Read the model definition and answer for the solid it produces. Units are mm, in the model's axes. A direction names the side the tool comes from. Coordinates: 2 decimals unless noted, no trailing zeros. Loops run counter-clockwise (first coordinate to the right, second up) from the corner with the lowest first, then second, coordinate; pieces in that order, holes last. Notation, with made-up numbers: M 51,-31 L 110,-31 A31 ccw 110,-5 Z; hole C 81,-32 d6. An arc over 180 degrees is marked long. Put each result on its own line as item: value.
from build123d import *

# Parameters (mm, degrees)
BOSS_EXTRUDE1_DEPTH     = 3.175
SKETCH2_R               = 19.9
CUT_EXTRUDE1_DEPTH      = 140.49939292
ESQUISSE2_R             = 1.5
ENL_V_MAT_EXTRU_1_DEPTH = 140.49939292
SKETCH5_R               = 1.625
CUT_EXTRUDE3_DEPTH      = 140.49939292
CUT_EXTRUDE4_DEPTH      = 140.49939292


with BuildPart() as part:
    # Sketch1 → Boss-Extrude1 (new body)
    with BuildSketch(Plane(origin=(0, 0, 0), x_dir=(1, 0, 0), z_dir=(0, 1, 0))):
        with BuildLine():
            Line((-27.5, -100), (-34.975254116, 98.684097441))
            ThreePointArc((-34.975254116, 98.684097441), (0, 135), (34.975254116, 98.684097441))
            Line((34.975254116, 98.684097441), (27.5, -100))
            ThreePointArc((27.5, -100), (0, -127.5), (-27.5, -100))
        make_face()
    extrude(amount=BOSS_EXTRUDE1_DEPTH)

    # Sketch2 → Cut-Extrude1 (cut, through all)
    with BuildSketch(Plane(origin=(0, 3.175, 0), x_dir=(1, 0, 0), z_dir=(0, 1, 0))):
        with Locations(Location((0, -100, 0), (0, 0, 270))):
            Circle(SKETCH2_R)
        with Locations(Location((0, 100, 0), (0, 0, 270))):
            Circle(SKETCH2_R)
    extrude(amount=-CUT_EXTRUDE1_DEPTH, mode=Mode.SUBTRACT)

    # Esquisse2 → Enlèv. mat.-Extru.1 (cut, through all)
    with BuildSketch(Plane(origin=(0, 3.175, 0), x_dir=(1, 0, 0), z_dir=(0, 1, 0))):
        with Locations(Location((19.339370465, 80.660629535, 0), (0, 0, 270))):
            Circle(ESQUISSE2_R)
        with Locations(Location((19.339370465, 119.339370465, 0), (0, 0, 270))):
            Circle(ESQUISSE2_R)
        with Locations(Location((-19.339370465, 119.339370465, 0), (0, 0, 270))):
            Circle(ESQUISSE2_R)
        with Locations(Location((-19.339370465, 80.660629535, 0), (0, 0, 270))):
            Circle(ESQUISSE2_R)
    extrude(amount=-ENL_V_MAT_EXTRU_1_DEPTH, mode=Mode.SUBTRACT)

    # Sketch5 → Cut-Extrude3 (cut, through all)
    with BuildSketch(Plane(origin=(0, 3.175, 0), x_dir=(1, 0, 0), z_dir=(0, 1, 0))):
        with Locations(Location((-27.256476824, 42.340455159, 0), (0, 0, 270))):
            Circle(SKETCH5_R)
        with Locations(Location((-26.241351992, 15.359544841, 0), (0, 0, 270))):
            Circle(SKETCH5_R)
        with Locations(Location((26.241351992, 15.359544841, 0), (0, 0, 270))):
            Circle(SKETCH5_R)
        with Locations(Location((27.256476824, 42.340455159, 0), (0, 0, 270))):
            Circle(SKETCH5_R)
        Polygon((-21.15, 45.828069991), (-16.978069991, 50), (16.978069991, 50), (21.15, 45.828069991), (21.15, 11.871930009), (16.978069991, 7.7), (-16.978069991, 7.7), (-21.15, 11.871930009), align=None)
    extrude(amount=-CUT_EXTRUDE3_DEPTH, mode=Mode.SUBTRACT)

    # Sketch7 → Cut-Extrude4 (cut, through all)
    with BuildSketch(Plane(origin=(0, 3.175, 0), x_dir=(1, 0, 0), z_dir=(0, 1, 0))):
        with BuildLine():
            Line((17.892039301, -34.947326615), (-12.749738424, -9.235822228))
            ThreePointArc((-12.749738424, -9.235822228), (-18.385066635, -9.728849561), (-17.892039301, -15.364177772))
            Line((-17.892039301, -15.364177772), (12.749738424, -41.07568216))
            ThreePointArc((12.749738424, -41.07568216), (18.385066635, -40.582654826), (17.892039301, -34.947326615))
        make_face()
    extrude(amount=-CUT_EXTRUDE4_DEPTH, mode=Mode.SUBTRACT)


solid = part.part
1) Find section B-B, the plane z = 12.3. Write down the section's boundary in (x, y) (3 decimals), plus the area to 3 significant figures.
Answer list:
outline: M -30.8,0 L -19.321,0 L -19.321,3.175 L -30.8,3.175 Z; M -9.098,0 L 30.8,0 L 30.8,3.175 L -9.098,3.175 Z
area: 163 mm^2
2) Which of the six approach directions +Z, -Z, +X, -X, +Y, -Y give full straight-line access (tool end or side, diameter ignored) to faces 1 (the flat face through (-2.786, 1.61, 28.04)), 2 (the flat face through (-31.185, 1.565, 2.049))?
Answer list:
face 1: +Y, -Y
face 2: +Z, -X, +Y, -Y
3) Find section A-A, the plane x = 0. Write down the section's boundary in (y, z) (3 decimals).
Answer list:
outline: M 0,-135 L 3.175,-135 L 3.175,-119.9 L 0,-119.9 Z; M 0,-80.1 L 3.175,-80.1 L 3.175,-50 L 0,-50 Z; M 0,-7.7 L 3.175,-7.7 L 3.175,19.934 L 0,19.934 Z; M 0,30.377 L 3.175,30.377 L 3.175,80.1 L 0,80.1 Z; M 0,119.9 L 3.175,119.9 L 3.175,127.5 L 0,127.5 Z
4) Straight lines are drawn through the part: line 1 (Z direction, x = -9, y = 0.9); line 2 (Z direction, x = -11, y = 1.65); line 3 (X direction, y = 2.45, z = 100). For each, find the intervals that lie inside material, in ascending order. Write a range as [from, to].
Answer list:
line 1: z = [-133.82, -117.75], [-82.25, -50], [-7.7, 12.38], [22.83, 82.25], [117.75, 125.99]
line 2: z = [-133.23, -116.58], [-83.42, -50], [-7.7, 10.7], [21.15, 83.42], [116.58, 125.2]
line 3: x = [-27.5, -19.9], [19.9, 27.5]
5) Find section D-D, the plane z = -29. Write down the section's boundary in (x, y) (3 decimals).
Answer list:
outline: M -32.353,0 L -21.15,0 L -21.15,3.175 L -32.353,3.175 Z; M 21.15,0 L 32.353,0 L 32.353,3.175 L 21.15,3.175 Z
6) Given pin 1 Ø1.6 at (y, z) = (1, -35) entering from -X; pin 2 Ø1 at (y, z) = (1, -97.5) entering from -X; pin 3 Ø1 at (y, z) = (2, -65.5) entering from -X, each flat-ended and moving along its own axis, determine where each tip first touches the part or whether it passes through.
Answer list:
pin 1: stops at x = -32.61
pin 2: stops at x = -34.95
pin 3: stops at x = -33.75
7) Find section C-C, the plane y = 1.45. Count the separate pieces of the cut face and the enclosed holes in it, plus the area to 3 significant figures.
Answer list:
separate pieces: 1
enclosed holes: 12
area: 10,900 mm^2
8) Determine the mould class of faces 3 (the flat face through (31.29, 1.57, -0.73)), 4 (the cylindrical face through (-12.1, 1.6, 84.2)), 5 (the flat face through (0, 3.175, -6)) for opening direction X: released by +X, released by -X, zero draft, split by the parting line, or undercut.
Answer list:
face 3: released by +X
face 4: undercut
face 5: zero draft
